Could you check a few things on this model? Use its own coordinates, in mm. A direction names the side the tool comes from. Round coordinates to 2 decimals unless told otherwise and drop trailing zeros. Order: outer loops, then holes, each group sorted by start corner. A loop starts at its lowest first (then second) coordinate and runs counter-clockwise, first axis right, second up. Notation, with made-up numbers: M -22.75,70.25 L 36.25,70.25 A22 ccw 36.25,91.25 Z; hole C 48.5,57 d9. An arc over 180 degrees is marked long. Write each question's results on one line, items separated by ' | '. Start each with the question number.
1. Suppose I cut it at B-B on y = 8.25. Write out the boundary of the cut face in (x, z).
2. We'd pull the mould along X, two halves only. Please class faces 6 (the cylindrical face through (-24.695, 15.436, -11.493)), 7 (the flat face through (1, 5, -16)), 8 (the flat face through (37.31, 19.92, 27.46)): released by +X, released by -X, zero draft, split by the parting line, or undercut.
3. Suppose I cut it at C-C on x = 22. Write out the boundary of the cut face in (y, z).
4. I'm going to push flat-ended pins straight in: pin 1 (5 mm diameter, centred on x = -16.5, y = 21, fed in from +Z); pin 2 (0.8 mm diameter, centred on x = 50.5, y = 18.5, fed in from +Z); pin 3 (4 mm diameter, centred on x = 2, y = 18, fed in from -Z). Where does each tip first touch, or does it pass through?
5. For faces 1 (the cylindrical face through (26.01, 10.59, 24.51)), 2 (the flat face through (0, 18, 28)), 3 (the flat face through (49, 18, -14)), 4 (the cylindrical face through (0.9, 14, -15.9)), 5 (the flat face through (35, 5, 35)), which set-ups out of +Z, -Z, +X, -X, +Y, -Y let a thin tool reach every point of the face, with its end or its side?
6. Suppose I cut it at A-A on z = 35. Write out the boundary of the cut face in (x, y), and give its area (3 significant figures).
7. Suppose I cut it at D-D on x = -10.5. Write out the boundary of the cut face in (y, z), and give its area (3 significant figures).
8. Please list where these lines run through material, in increasing order: L1, parallel to X at y = 3.25, z = 35; L2, parallel to Z at x = 3, y = 2; L3, parallel to X at y = 2.25, z = 12.5.
from build123d import *

# Parameters (mm, degrees)
SKETCH_1_5_W             = 10
SKETCH_1_5_H             = 10
SKETCH_1_5_R             = 2.1
EXTRUDE_4_DEPTH          = 10
EXTRUDE_4_2_DEPTH        = 10
SKETCH_1_6_W             = 10
SKETCH_1_6_H             = 10
SKETCH_1_6_R             = 2.1
EXTRUDE_5_DEPTH          = 35
SKETCH_1_W               = 20
SKETCH_1_H               = 35
EXTRUDE_7_DEPTH          = 19
SKETCH_1_W_2             = 22
EXTRUDE_7_2_DEPTH        = 19
FILLET_8_SIZE            = 3
FILLET_9_SIZE            = 3
EXTRUDE_8_DEPTH          = 18
SKETCH_2_W               = 37
SKETCH_2_H               = 30
CUT_EXTRUDE_2_DEPTH      = 138.800580637
CUT_EXTRUDE_3_DEPTH      = 113.111551644
CUT_EXTRUDE_3_DEPTH_BACK = 113.111551644
CUT_EXTRUDE_4_DEPTH      = 6
CUT_EXTRUDE_START        = -5.5
CUT_EXTRUDE_5_DEPTH      = 5.5
EXTRUDE_START            = 24
EXTRUDE_14_DEPTH         = 6
EXTRUDE_15_DEPTH         = 5
CUT_EXTRUDE_6_DEPTH      = 138.800580637
CUT_EXTRUDE_6_DEPTH_BACK = 138.800580637
EXTRUDE_START_2          = -2
SKETCH_10_R              = 4.1
EXTRUDE_17_DEPTH         = 2
SKETCH_11_R              = 4.1
EXTRUDE_18_DEPTH         = 1.5
EXTRUDE_19_DEPTH         = 6
CUT_EXTRUDE_7_DEPTH      = 36
CUT_EXTRUDE_7_DEPTH_BACK = 1
EXTRUDE_START_3          = 3
SKETCH_13_R              = 12
SKETCH_13_R_2            = 4.1
EXTRUDE_20_DEPTH         = 3
CUT_EXTRUDE_9_DEPTH      = 40


with BuildPart() as part:
    # Sketch 1_5 → Extrude 4 (new body)
    with BuildSketch(Plane(origin=(0, 0, 0), x_dir=(1, 0, 0), z_dir=(0, 1, 0))):
        with Locations((-40, -35)):
            Rectangle(SKETCH_1_5_W, SKETCH_1_5_H)
        with Locations(Location((-40, -35, 0), (0, 0, 270))):
            Circle(SKETCH_1_5_R, mode=Mode.SUBTRACT)
    extrude(amount=EXTRUDE_4_DEPTH)



with BuildPart() as body_2:
    # Sketch 1_5 → Extrude 4 2 (new body)
    with BuildSketch(Plane(origin=(0, 0, 0), x_dir=(1, 0, 0), z_dir=(0, 1, 0))):
        with Locations((40, -35)):
            Rectangle(SKETCH_1_5_W, SKETCH_1_5_H)
        with Locations(Location((40, -35, 0), (0, 0, 270))):
            Circle(SKETCH_1_5_R, mode=Mode.SUBTRACT)
    extrude(amount=EXTRUDE_4_2_DEPTH)


with BuildPart() as body_3:
    # Sketch 1_6 → Extrude 5 (new body)
    # profile 1 of 3: a face of its own
    with BuildSketch(Plane(origin=(0, 0, 0), x_dir=(1, 0, 0), z_dir=(0, 1, 0))):
        Polygon((45, 48), (35, 48), (-35, 48), (-45, 48), (-60, 48), (-60, 43), (-60, 16), (-55, 16), (-55, 43), (55, 43), (55, 16), (60, 16), (60, 43), (60, 48), align=None)
    # profile 2 of 3: a face of its own
    with BuildSketch(Plane(origin=(0, 0, 0), x_dir=(1, 0, 0), z_dir=(0, 1, 0))):
        with Locations((-40, 53)):
            Rectangle(SKETCH_1_6_W, SKETCH_1_6_H)
        with Locations(Location((-40, 53, 0), (0, 0, 270))):
            Circle(SKETCH_1_6_R, mode=Mode.SUBTRACT)
    # profile 3 of 3: a face of its own
    with BuildSketch(Plane(origin=(0, 0, 0), x_dir=(1, 0, 0), z_dir=(0, 1, 0))):
        with Locations((40, 53)):
            Rectangle(SKETCH_1_6_W, SKETCH_1_6_H)
        with Locations(Location((40, 53, 0), (0, 0, 270))):
            Circle(SKETCH_1_6_R, mode=Mode.SUBTRACT)
    extrude(amount=EXTRUDE_5_DEPTH)


with BuildPart() as body_4:
    # Sketch 1 → Extrude 7 (new body)
    with BuildSketch(Plane(origin=(0, 0, 0), x_dir=(1, 0, 0), z_dir=(0, 1, 0))):
        with Locations((50, -6.5)):
            Rectangle(SKETCH_1_W, SKETCH_1_H)
    extrude(amount=EXTRUDE_7_DEPTH)

    # Fillet 9
    # a fillet whose section is not a circle: 3 mm, written as the material it takes off along each edge
    with BuildSketch(Plane(origin=(40, 19, 31.5), x_dir=(0, -1, 0), z_dir=(0, 0, -1)), Plane(origin=(60, 19, -18.5), x_dir=(0, -1, 0), z_dir=(0, 0, 1))) as fillet_9_piece_1:
        with BuildLine():
            Bezier((FILLET_9_SIZE, 0), (0, 0), (0, -FILLET_9_SIZE), weights=[1, 1, 1])
            Line((0, -FILLET_9_SIZE), (0, 0))
            Line((0, 0), (FILLET_9_SIZE, 0))
        make_face()
    extrude(amount=50, mode=Mode.SUBTRACT)


with BuildPart() as body_5:
    # Sketch 1 → Extrude 7 2 (new body)
    with BuildSketch(Plane(origin=(0, 0, 0), x_dir=(1, 0, 0), z_dir=(0, 1, 0))):
        with Locations((-49, -6.5)):
            Rectangle(SKETCH_1_W_2, SKETCH_1_H)
    extrude(amount=EXTRUDE_7_2_DEPTH)

    # Fillet 8
    # a fillet whose section is not a circle: 3 mm, written as the material it takes off along each edge
    with BuildSketch(Plane(origin=(-60, 19, -18.5), x_dir=(0, -1, 0), z_dir=(0, 0, 1)), Plane(origin=(-38, 19, 31.5), x_dir=(0, -1, 0), z_dir=(0, 0, -1))) as fillet_8_piece_1:
        with BuildLine():
            Bezier((FILLET_8_SIZE, 0), (0, 0), (0, FILLET_8_SIZE), weights=[1, 1, 1])
            Line((0, FILLET_8_SIZE), (0, 0))
            Line((0, 0), (FILLET_8_SIZE, 0))
        make_face()
    extrude(amount=50, mode=Mode.SUBTRACT)


with BuildPart() as part_1:
    add(part.part)

    add(body_2.part)  # Extrude 8 merges body 2

    add(body_3.part)  # Extrude 8 merges body 3

    add(body_4.part)  # Extrude 8 merges body 4

    add(body_5.part)  # Extrude 8 merges body 5
    # Sketch 1_9 → Extrude 8 (add)
    with BuildSketch(Plane(origin=(0, 0, 0), x_dir=(1, 0, 0), z_dir=(0, 1, 0))):
        Polygon((-38, 11), (40, 11), (60, 11), (60, 16), (55, 16), (-55, 16), (-60, 16), (-60, 11), align=None)
        Polygon((40, -24), (60, -24), (60, -30), (45, -30), (35, -30), (-35, -30), (-45, -30), (-60, -30), (-60, -24), (-38, -24), align=None)
    extrude(amount=EXTRUDE_8_DEPTH)

    # Sketch 2 → Cut-Extrude 2 (cut, through all)
    with BuildSketch(Plane.ZY.offset(60)):
        with Locations((-39.5, 15)):
            Rectangle(SKETCH_2_W, SKETCH_2_H)
    extrude(amount=-CUT_EXTRUDE_2_DEPTH, mode=Mode.SUBTRACT)

    # Sketch 3 → Cut-Extrude 3 (cut, two sides: drawn at the far end of the back side and taken through both)
    with BuildSketch(Plane.XY.offset(30).offset(-CUT_EXTRUDE_3_DEPTH_BACK)):
        with BuildLine():
            Line((-4.1, 18), (4.1, 18))
            ThreePointArc((4.1, 18), (0, 13.9), (-4.1, 18))
        make_face()
    extrude(amount=CUT_EXTRUDE_3_DEPTH + CUT_EXTRUDE_3_DEPTH_BACK, mode=Mode.SUBTRACT)

    # Sketch 6 → Cut-Extrude 4 (cut)
    with BuildSketch(Plane(origin=(0, 0, -16), x_dir=(-1, 0, 0), z_dir=(0, 0, -1))):
        with BuildLine():
            Line((-26.264911064, 18), (-23.735088936, 18))
            ThreePointArc((-23.735088936, 18), (-25, 17.8), (-26.264911064, 18))
        make_face()
        with BuildLine():
            Line((23.803098267, 18), (26.13923016, 18))
            ThreePointArc((26.13923016, 18), (24.971164214, 17.830091849), (23.803098267, 18))
        make_face()
    extrude(amount=-CUT_EXTRUDE_4_DEPTH, mode=Mode.SUBTRACT)

    # Sketch 7 → Cut-Extrude 5 (cut)
    with BuildSketch(Plane.XY.offset(30).offset(CUT_EXTRUDE_START)):
        with BuildLine():
            Line((-26.13923016, 18), (-23.803098267, 18))
            ThreePointArc((-23.803098267, 18), (-24.971164214, 17.830091849), (-26.13923016, 18))
        make_face()
        with BuildLine():
            Line((23.735088936, 18), (26.264911064, 18))
            ThreePointArc((26.264911064, 18), (25, 17.8), (23.735088936, 18))
        make_face()
    extrude(amount=CUT_EXTRUDE_5_DEPTH, mode=Mode.SUBTRACT)

    # Extrude 14: read off the stored shape, not the designer's step
    # Extrude 14 outline → Extrude 14 (add)
    with BuildSketch(Plane.XY.offset(EXTRUDE_START)):
        with BuildLine():
            ThreePointArc((23.735088935, 18), (21.68366653, 19.489205044), (20.9, 21.9))
            Line((20.9, 21.9), (4.1, 18))
            Line((4.1, 18), (23.735088935, 18))
        make_face()
        with BuildLine():
            ThreePointArc((-20.9, 21.9), (-21.711099928, 19.473259749), (-23.803098267, 18))
            Line((-23.803098267, 18), (-4.1, 18))
            Line((-4.1, 18), (-20.9, 21.9))
        make_face()
        with BuildLine():
            ThreePointArc((-26.13923016, 18), (-28.265749222, 19.45947321), (-29.1, 21.9))
            Line((-29.1, 21.9), (-40, 18))
            Line((-40, 18), (-26.13923016, 18))
        make_face()
    extrude(amount=EXTRUDE_14_DEPTH)

    # Sketch 6_6 → Extrude 15 (add)
    with BuildSketch(Plane(origin=(0, 0, -16), x_dir=(-1, 0, 0), z_dir=(0, 0, -1))):
        with BuildLine():
            ThreePointArc((-23.735088936, 18), (-21.68366653, 19.489205044), (-20.9, 21.9))
            Line((-20.9, 21.9), (-4.1, 18))
            Line((-4.1, 18), (-23.735088936, 18))
        make_face()
        with BuildLine():
            ThreePointArc((20.9, 21.9), (21.711099928, 19.473259749), (23.803098267, 18))
            Line((23.803098267, 18), (4.1, 18))
            Line((4.1, 18), (20.9, 21.9))
        make_face()
        with BuildLine():
            Line((29.042328427, 21.9), (40, 18))
            Line((40, 18), (26.13923016, 18))
            ThreePointArc((26.13923016, 18), (28.2312285, 19.473259749), (29.042328427, 21.9))
        make_face()
        with BuildLine():
            Line((-38, 18), (-26.264911064, 18))
            ThreePointArc((-26.264911064, 18), (-28.31633347, 19.489205044), (-29.1, 21.9))
            Line((-29.1, 21.9), (-38, 18))
        make_face()
    extrude(amount=-EXTRUDE_15_DEPTH)

    # Sketch 9 → Cut-Extrude 6 (cut, two sides: drawn at the far end of the back side and taken through both)
    with BuildSketch(Plane.ZY.offset(60).offset(-CUT_EXTRUDE_6_DEPTH_BACK)):
        Polygon((-58, 34.891965128), (-58, 35), (-16, 35), (-16, 34.9), align=None)
    extrude(amount=CUT_EXTRUDE_6_DEPTH + CUT_EXTRUDE_6_DEPTH_BACK, mode=Mode.SUBTRACT)

    # Sketch 10 → Extrude 17 (add)
    with BuildSketch(Plane.XY.offset(30).offset(EXTRUDE_START_2)):
        with Locations((25, 21.9)):
            Circle(SKETCH_10_R)
        with Locations((0, 18)):
            Circle(SKETCH_10_R)
        with Locations((-32.5, 21.9)):
            Circle(SKETCH_10_R)
    extrude(amount=EXTRUDE_17_DEPTH)

    # Sketch 11 → Extrude 18 (add)
    with BuildSketch(Plane(origin=(0, 0, -16), x_dir=(-1, 0, 0), z_dir=(0, 0, -1))):
        with Locations((-25, 21.9)):
            Circle(SKETCH_11_R)
        with Locations((32.5, 21.9)):
            Circle(SKETCH_11_R)
    extrude(amount=-EXTRUDE_18_DEPTH)

    # Extrude 19: read off the stored shape, not the designer's step
    # Extrude 19 outline → Extrude 19 (add)
    with BuildSketch(Plane.XY.offset(EXTRUDE_START)):
        with BuildLine():
            Line((26.264911064, 18), (38, 18))
            Line((38, 18), (36.6, 21.9))
            ThreePointArc((36.6, 21.9), (31.478486585, 19.828016661), (26.264911064, 18))
        make_face()
    extrude(amount=EXTRUDE_19_DEPTH)

    # Sketch 12 → Cut-Extrude 7 (cut, two sides: drawn at the far end of the back side and taken through both)
    with BuildSketch(Plane(origin=(0, 0, 24), x_dir=(-1, 0, 0), z_dir=(0, 0, -1)).offset(-CUT_EXTRUDE_7_DEPTH_BACK)):
        with BuildLine():
            Line((-40, 0), (-40, 18))
            Line((-40, 18), (-38, 18))
            Line((-38, 18), (-36.331975313, 22.6466402))
            ThreePointArc((-36.331975313, 22.6466402), (-26.202477843, 10.607295137), (-13.76489452, 20.243636228))
            Line((-13.76489452, 20.243636228), (-6.476544564, 18.551697845))
            ThreePointArc((-6.476544564, 18.551697845), (0, 11.5), (6.476544564, 18.551697845))
            Line((6.476544564, 18.551697845), (18.497791598, 21.342344478))
            ThreePointArc((18.497791598, 21.342344478), (24.835126866, 15.431515556), (31.414269621, 21.071958576))
            Line((31.414269621, 21.071958576), (38, 18.71559633))
            Line((38, 18.71559633), (38, 0))
            Line((38, 0), (-40, 0))
        make_face()
    extrude(amount=CUT_EXTRUDE_7_DEPTH + CUT_EXTRUDE_7_DEPTH_BACK, mode=Mode.SUBTRACT)

    # Sketch 13 → Extrude 20 (add)
    with BuildSketch(Plane(origin=(0, 0, -16), x_dir=(-1, 0, 0), z_dir=(0, 0, -1)).offset(EXTRUDE_START_3)):
        with Locations(Location((0, 18, 0), (0, 0, 171.361826288))):
            Circle(SKETCH_13_R)
        with Locations((0, 18)):
            Circle(SKETCH_13_R_2, mode=Mode.SUBTRACT)
    extrude(amount=-EXTRUDE_20_DEPTH)

    # Sketch 14 → Cut-Extrude 9 (cut)
    with BuildSketch(Plane(origin=(0, 0, 0), x_dir=(-1, 0, 0), z_dir=(0, -1, 0))):
        Polygon((-55, 16), (-55, 43), (55, 43), (55, 16), (60, 16), (60, 63), (-60, 63), (-60, 16), align=None)
    extrude(amount=-CUT_EXTRUDE_9_DEPTH, mode=Mode.SUBTRACT)


solid = part_1.part
Filled sheet:
1) outline: M -60,-16 L -7,-16 L -7,-19 L 7,-19 L 7,-16 L 60,-16 L 60,30 L 45,30 L 45,40 L 35,40 L 35,30 L -35,30 L -35,40 L -45,40 L -45,30 L -60,30 Z; hole C -40,35 d4.2; hole M -38,-12 L 40,-12 L 40,25 L -38,25 Z; hole C 40,35 d4.2
2) face 6: undercut | face 7: zero draft | face 8: released by +X
3) outline: M 0,-16 L 24.69,-16 L 24.69,-14.5 L 19.11,-14.5 L 19.11,-11 L 10.95,-11 L 10.95,-12 L 0,-12 Z; M 0,25 L 10.95,25 L 10.95,24 L 19.11,24 L 19.11,28 L 24.69,28 L 24.69,30 L 0,30 Z
4) pin 1: stops at z = 30 | pin 2: stops at z = 24 | pin 3: stops at z = 28
5) face 1: -Y | face 2: -Z, +Y | face 3: -Z, +X, +Y | face 4: -Z | face 5: +Z, +Y, -Y
6) outline: M -45,0 L -42.1,0 L -42.1,10 L -45,10 Z; M -37.9,0 L -35,0 L -35,10 L -37.9,10 Z; M 35,0 L 37.9,0 L 37.9,10 L 35,10 Z; M 42.1,0 L 45,0 L 45,10 L 42.1,10 Z | area: 116 mm^2
7) outline: M 0,-16 L 12.19,-16 L 12.19,-19 L 23.81,-19 L 23.81,-16 L 19.49,-16 L 19.49,-12 L 0,-12 Z; M 0,25 L 19.49,25 L 19.49,30 L 0,30 Z | area: 210 mm^2
8) L1: x = -45 to -42.1, -37.9 to -35, 35 to 37.9, 42.1 to 45 | L2: z = -16 to -12, 25 to 30 | L3: x = -60 to -38, 40 to 60
